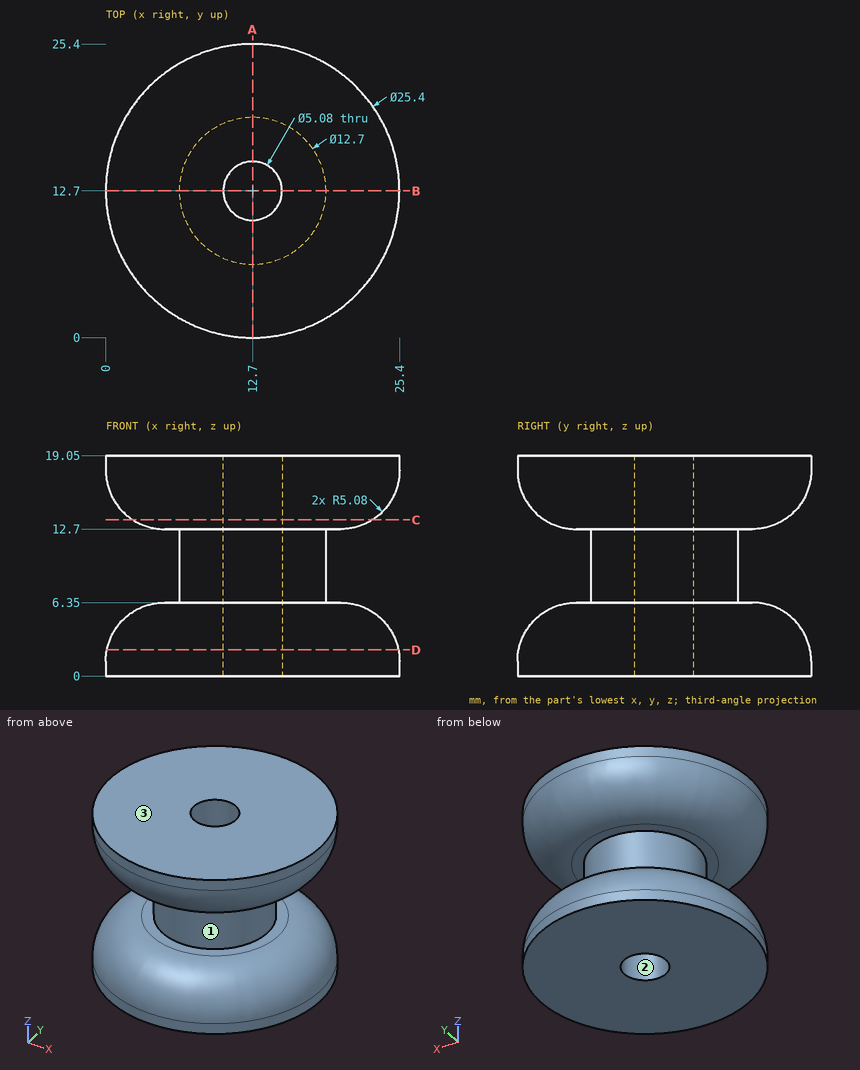
Print and shaded views of the part. All mm, measured from the part's lowest x, y and z. Round coordinates to 2 decimals unless told otherwise and drop trailing zeros. Write each loop counter-clockwise with the first axis right and the second up, starting at its lowest first coordinate (ties: lowest second). Pieces come first, ordered by that corner, then holes. Notation, with made-up numbers: (3, -4) -> (41, -4) arc R4 cw to (41, 2) -> close; hole circle Ø11 at (74.25, -6.75). An arc over 180 degrees is marked (long way). Return JSON: item names as keys, results as strings. Group by question number.
Q1. Mould opens along X. For the marked faces 1, 2 and 3 say: pulls with the +X half, pulls with the -X half, needs draft (parallel to the pull), parting line crosses it, or undercut.
Q2. Saw through at D-D on z = 2.25. Write the cut outline in (x, y).
Q3. Saw through at A-A on x = 12.7. Write the cut outline in (y, z), plus the area to 3 significant figures.
Q4. Pin check, flat tips, straight feed: pin 1 (1.5 mm diameter, centred on x = 15.5, z = 9.5, fed in from +Y); pin 2 (6 mm diameter, centred on y = 18.5, z = 3.5, fed in from +X); pin 3 (2 mm diameter, centred on x = 20.5, z = 13.5, fed in from -Y); pin 4 (3 mm diameter, centred on y = 3.5, z = 9, fed in from -X) (3 decimals). Stop position of each tip, or through.
Q5. Probe L1, parallel to Y at x = 12.7, z = 10; L2, parallel to Z at x = 19.25, y = 16.25. List the from-to ranges inside material, lowest first. Write a range as [from, to].
Q6. Saw through at C-C on z = 13.5. Write the cut outline in (x, y).
Answer:
{
 "1": {"face 1": "parting line crosses it", "face 2": "undercut", "face 3": "needs draft"},
 "2": {"outline": "circle Ø25.21 at (12.7, 12.7); hole circle Ø5.08 at (12.7, 12.7)"},
 "3": {"outline": "(0, 0) -> (10.16, 0) -> (10.16, 19.05) -> (0, 19.05) -> (0, 17.78) arc R5.08 ccw to (5.08, 12.7) -> (6.35, 12.7) -> (6.35, 6.35) -> (5.08, 6.35) arc R5.08 ccw to (0, 1.27) -> close; (15.24, 0) -> (25.4, 0) -> (25.4, 1.27) arc R5.08 ccw to (20.32, 6.35) -> (19.05, 6.35) -> (19.05, 12.7) -> (20.32, 12.7) arc R5.08 ccw to (25.4, 17.78) -> (25.4, 19.05) -> (15.24, 19.05) -> close", "area": "284 mm2"},
 "4": {"pin 1": "y = 18.71", "pin 2": "x = 24.94", "pin 3": "y = 3.96", "pin 4": "through"},
 "5": {"L1": "[6.35, 10.16], [15.24, 19.05]", "L2": "[0, 6.35], [12.7, 19.05]"},
 "6": {"outline": "circle Ø20.71 at (12.7, 12.7); hole circle Ø5.08 at (12.7, 12.7)"}
}
